Input: part model. Units: mm. Frame: model coordinates. Coordinates: 2 decimals unless noted, no trailing zeros. Order: outer loops, then holes, each group sorted by start corner. A loop starts at its lowest first (then second) coordinate and runs counter-clockwise, first axis right, second up. Notation, with made-up numbers: (35.25, -34.75) -> (52.25, -34.75) arc R22 ccw to (52.25, -21.75) -> close; hole circle Ø3 at (-7, -11). An arc over 180 degrees is marked (long way). Use CSV: the item, a comma, the result in double quotes. Start each with the question number.
Autodesk Inventor part; units mm, degrees
ref_plane "YZ Plane" through (0, 0, 0) normal (1, 0, 0) x (0, 1, 0)
ref_plane "XZ Plane" through (0, 0, 0) normal (0, 1, 0) x (-1, 0, 0)
ref_plane "XY Plane" through (0, 0, 0) normal (0, 0, 1) x (1, 0, 0)
sketch "Sketch1" plane through (0, 0, 0) normal (0, 0, 1) x (1, 0, 0)
  line L0 (-1177.925, -1219.2) -> (1177.925, -1219.2)
  line L1 (1177.925, -1219.2) -> (1177.925, 1219.2)
  line L2 (1177.925, 1219.2) -> (-1177.925, 1219.2)
  line L3 (-1177.925, 1219.2) -> (-1177.925, -1219.2)
  line L4 (-1177.925, -1219.2) -> (1177.925, 1219.2) construction
  line L5 (1177.925, -1219.2) -> (-1177.925, 1219.2) construction
  line L6 (-1177.925, -1219.2) -> (-307.975, -1219.2)
  line L7 (-307.975, -1219.2) -> (-307.975, 1219.2)
  line L8 (1177.925, 1219.2) -> (-307.975, -1219.2)
  line L9 (-1177.925, 1219.2) -> (-307.975, -1219.2)
  line L10 (-345.9327, -1196.0695) -> (-270.0173, -1242.3305)
  line L11 (-349.8404, -1234.1363) -> (-266.1096, -1204.2637)
  line L12 (-1219.7904, 1204.2637) -> (-1136.0596, 1234.1363)
  line L13 (1215.8827, 1196.0695) -> (1139.9673, 1242.3305)
  line L14 (1139.9673, 1242.3305) -> (-345.9327, -1196.0695)
  line L15 (-270.0173, -1242.3305) -> (1215.8827, 1196.0695)
  line L16 (-266.1096, -1204.2637) -> (-1136.0596, 1234.1363)
  line L17 (-1219.7904, 1204.2637) -> (-349.8404, -1234.1363)
  point P0 (0, 0)
  point P1 (-307.975, -1086.9184)
  point P2 (-1130.7308, 1219.2)
  point P3 (-1177.925, 1086.9184)
  point P4 (-355.1692, -1219.2)
  point P5 (-307.975, -1219.2)
  point P6 (-307.975, -1133.78)
  point P7 (1125.8722, 1219.2)
  point P8 (-255.9222, -1219.2)
  point P9 (1177.925, 1133.78)
  dimension "d0" = 2355.85
  dimension "d1" = 2438.4
  dimension "d2" = 869.95
  dimension "d3" = 88.9
  dimension "d4" = 88.9
  dimension "d6" = 88.9
  dimension "d7" = 88.9
extrude "Extrusion1" add sketch "Sketch1" along normal blind 38.1 contours L11 L16 L8 L1 L15 L0 | L7 L14 L16 L8 | L8 L16 L11 | L16 L14 L2 L8
properties part number "S_2x4x112.420"
1. Section A-A on z = 26. Return loops of the section in (x, y) (3 decimals).
2. Section B-B on y = -438. Return loops of the section in (x, z).
3. Pull-direction query (X, two-part tool) for faces 1 (the face through (418.986, 59.181, 18.783)), 2 (the face through (450.964, -59.181, 18.783)), 3 (the face through (432, 6, 38.1)); classes: released by +X, released by -X, zero draft, split by the parting line, or undercut.
4. Section C-C on x = -109. Return loops of the section in (y, z), then the cut area to 3 significant figures.
5. Material intervals for line 1 along X through (y, z) = (-719.5, 14); line 2 along Y through (x, z) = (626, 11); line 3 along Y through (x, z) = (208.5, 26.5), sorted ascending.
6. Contact query for flat-ended pins moving along their axis: P1, Ø12, axis at y = -68.5, z = 23.5, coming from the +X side; P2, Ø2, axis at x = 586.5, z = 5, coming from the -Y side; P3, Ø10, axis at y = 564, z = 9.5, coming from the -X side. Output: stop coordinate, or through.
Values follow:
1,outline,"(-307.975, -1219.2) -> (-255.922, -1219.2) -> (1177.925, 1133.78) -> (1177.925, 1219.2) -> (1125.872, 1219.2) -> (-307.975, -1133.78) -> close"
2,outline,"(116.02, 0) -> (220.12, 0) -> (220.12, 38.1) -> (116.02, 38.1) -> close"
3,face 1,"released by -X"
3,face 2,"released by +X"
3,face 3,"zero draft"
4,outline,"(-978.1, 0) -> (-807.26, 0) -> (-807.26, 38.1) -> (-978.1, 38.1) -> close"
4,area,"6,510 mm2"
5,line 1,"x = -55.52 to 48.58"
5,line 2,"y = 228.06 to 398.9"
5,line 3,"y = -457.07 to -286.23"
6,P1,"stops at x = 448.94"
6,P2,"stops at y = 161.6"
6,P3,"stops at x = 723.56"
